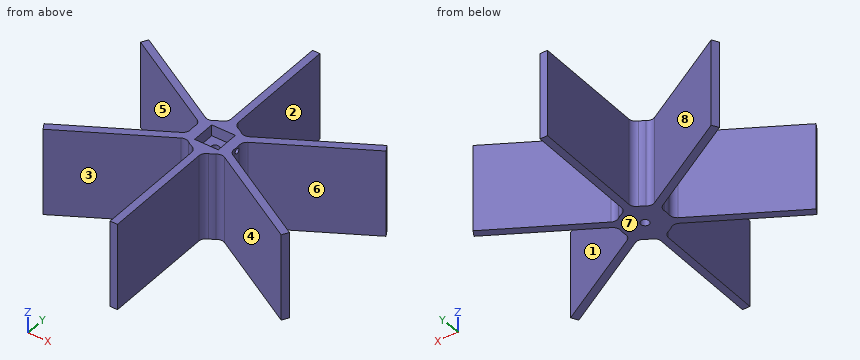
from build123d import *

# Parameters (mm, degrees)
BOSS_EXTRUDE1_DEPTH = 37.5
CIRPATTERN1_COUNT   = 6
FILLET1_R           = 6.35
SKETCH2_W           = 20.32
SKETCH2_H           = 20.32
CUT_EXTRUDE1_DEPTH  = 9.525
SKETCH3_R           = 3.571875
CUT_EXTRUDE2_DEPTH  = 173.631673961
SKETCH4_R           = 2.1828125
CUT_EXTRUDE3_DEPTH  = 171.784747264


with BuildPart() as part:
    # Sketch1 → Boss-Extrude1 (new, symmetric)
    with BuildSketch(Plane.XY):
        with BuildLine():
            Line((-3.175, 119.957990042), (-3.175, 18.783553311))
            ThreePointArc((-3.175, 18.783553311), (0, 19.05), (3.175, 18.783553311))
            Line((3.175, 18.783553311), (3.175, 119.957990042))
            Line((3.175, 119.957990042), (-3.175, 119.957990042))
        make_face()
        with BuildLine():
            Line((-3.175, 18.783553311), (-3.175, 0))
            Line((-3.175, 0), (3.175, 0))
            Line((3.175, 0), (3.175, 18.783553311))
            ThreePointArc((3.175, 18.783553311), (0, 19.05), (-3.175, 18.783553311))
        make_face()
        with BuildLine():
            Line((3.175, 0), (-3.175, 0))
            Line((-3.175, 0), (-3.175, 18.783553311))
            ThreePointArc((-3.175, 18.783553311), (-12.296722124, -14.549677831), (19.05, 0))
            ThreePointArc((19.05, 0), (14.549677831, 12.296722124), (3.175, 18.783553311))
            Line((3.175, 18.783553311), (3.175, 0))
        make_face()
    boss_extrude1 = extrude(amount=BOSS_EXTRUDE1_DEPTH, both=True)

    # CirPattern1: Boss-Extrude1 ×6 about axis
    cirpattern1_axis = Axis((0, 0, 0), (0, 0, 1))
    for i in range(1, CIRPATTERN1_COUNT):
        add(boss_extrude1.rotate(cirpattern1_axis, i * 360 / CIRPATTERN1_COUNT))

    # Fillet1
    fillet1_edges = [part.edges().sort_by_distance(p)[0] for p in [
        (14.679534341, 12.141407313, 0),
        (-17.854534341, 6.642145999, 0),
        (3.175, -18.783553311, 0),
        (17.854534341, -6.642145999, 0),
        (-14.679534341, -12.141407313, 0),
        (-14.679534341, 12.141407313, 0),
        (-3.175, -18.783553311, 0),
        (17.854534341, 6.642145999, 0),
        (14.679534341, -12.141407313, 0),
        (-17.854534341, -6.642145999, 0),
        (-3.175, 18.783553311, 0),
        (3.175, 18.783553311, 0),
    ]]
    fillet(fillet1_edges, radius=FILLET1_R)

    # Sketch2 → Cut-Extrude1 (cut)
    with BuildSketch(Plane.XY.offset(37.5)):
        Rectangle(SKETCH2_W, SKETCH2_H)
    extrude(amount=-CUT_EXTRUDE1_DEPTH, mode=Mode.SUBTRACT)

    # Sketch3 → Cut-Extrude2 (cut, through all)
    with BuildSketch(Plane.XY.offset(27.975)):
        Circle(SKETCH3_R)
    extrude(amount=-CUT_EXTRUDE2_DEPTH, mode=Mode.SUBTRACT)

    # Sketch4 → Cut-Extrude3 (cut, through all)
    with BuildSketch(Plane.ZY.offset(-10.16)):
        with Locations(Location((34.0075, 0, 0), (0, 0, 270))):
            Circle(SKETCH4_R)
    extrude(amount=-CUT_EXTRUDE3_DEPTH, mode=Mode.SUBTRACT)


solid = part.part
Geometry check sheet. Reference: the model listing, model coordinates, mm. Face numbers are marked on the shaded views. A direction names the side the tool comes from. Give positions to 0.01 mm unless a question says otherwise; leave off trailing zeros. Loops run counter-clockwise (first coordinate to the right, second up) from the corner with the lowest first, then second, coordinate; pieces in that order, holes last. Notation, with made-up numbers: (70.25, 30.5) -> (112.25, 30.5) arc R26 ccw to (112.25, 55.5) -> close; hole circle Ø8 at (12, 45). An arc over 180 degrees is marked (long way). Answer in a Markdown table with one row per item. Add a question column.
1) Material ranges on probe 1 along Z at (x, y) = (17, 0); probe 2 along Y at (x, z) = (0, 10.5); probe 3 along X at (y, z) = (59.5, -21.5) (3 decimals), recorded low to high. Write a range as from..to.
2) Cross-section at B-B on y = -34. Record the boundary of the cut face in (x, z) (3 decimals).
3) Gauge pin test, flat ends, axial feed: P1, Ø12, axis at y = -77, z = -25, coming from the -X side (3 decimals); P2, Ø4, axis at y = 0, z = 34.01, coming from the -X side; P3, Ø4.5, axis at x = 0, y = 0, coming from the -Z side; P4, Ø5, axis at y = -23, z = -27.5, coming from the +X side. Record the tip position at first contact, or that the pin passes through.
4) Draft check along Y on the marked faces 1, 2 and 3. Enter one of: pulls with the +Y half, pulls with the -Y half, needs draft (parallel to the pull), parting line crosses it, or undercut.
5) Cross-section at C-C on x = -77.5. Record the boundary of the cut face in (y, z).
6) Cross-section at A-A on x = 0. Record the boundary of the cut face in (y, z) (3 decimals), and give its area (3 significant figures).
7) Set-up check for the marked faces 4, 5, 6, 7 and 8: record each of +Z, -Z, +X, -X, +Y, -Y from which the full face is reachable in a straight line by a thin tool's end or side.
8) Cross-section at D-D on y = -83.5. Record the boundary of the cut face in (x, z) (3 decimals).
Outcome:
| question | item | result |
|---|---|---|
| 1 | probe 1 | z = -37.5..31.82, 36.19..37.5 |
| 1 | probe 2 | y = -119.96..-3.57, 3.57..119.96 |
| 1 | probe 3 | x = -104.163..-96.707, -3.175..3.175, 96.707..104.163 |
| 2 | outline | (-65.24, -37.5) -> (-52.54, -37.5) -> (-52.54, 37.5) -> (-65.24, 37.5) -> close; (-3.175, -37.5) -> (3.175, -37.5) -> (3.175, 37.5) -> (-3.175, 37.5) -> close; (52.54, -37.5) -> (65.24, -37.5) -> (65.24, 37.5) -> (52.54, 37.5) -> close |
| 3 | P1 | stops at x = -3.175 |
| 3 | P2 | stops at x = -19.05 |
| 3 | P3 | passes through |
| 3 | P4 | stops at x = 50.52 |
| 4 | face 1 | undercut |
| 4 | face 2 | needs draft |
| 4 | face 3 | pulls with the -Y half |
| 5 | outline | (-48.41, -37.5) -> (-41.08, -37.5) -> (-41.08, 37.5) -> (-48.41, 37.5) -> close; (41.08, -37.5) -> (48.41, -37.5) -> (48.41, 37.5) -> (41.08, 37.5) -> close |
| 6 | outline | (-119.958, -37.5) -> (-3.572, -37.5) -> (-3.572, 27.975) -> (-10.16, 27.975) -> (-10.16, 37.5) -> (-119.958, 37.5) -> close; (3.572, -37.5) -> (119.958, -37.5) -> (119.958, 37.5) -> (10.16, 37.5) -> (10.16, 27.975) -> (3.572, 27.975) -> close |
| 6 | area | 17,300 mm^2 |
| 7 | face 4 | +Z, -Z, -Y |
| 7 | face 5 | +Z, -Z, -X |
| 7 | face 6 | +Z, -Z, +X |
| 7 | face 7 | -Z, +X, -X, +Y, -Y |
| 7 | face 8 | +Z, -Z, +Y |
| 8 | outline | (-3.175, -37.5) -> (3.175, -37.5) -> (3.175, 37.5) -> (-3.175, 37.5) -> close |
